Part model, mm, in its own coordinate system. A direction names the side the tool comes from. Give positions to 0.01 mm unless a question says otherwise; leave off trailing zeros. Write each loop counter-clockwise with the first axis right and the second up, starting at its lowest first coordinate (ties: lowest second). Pieces come first, ordered by that corner, then holes.
from build123d import *

# Parameters (mm, degrees)
BOSS_EXTRUDE1_DEPTH = 9.525
SKETCH2_W           = 139.7
SKETCH2_H           = 25.4
CUT_EXTRUDE1_DEPTH  = 503.984538157


with BuildPart() as part:
    # Sketch1 → Boss-Extrude1 (new body)
    with BuildSketch(Plane.XY):
        with BuildLine():
            Line((25.4, 0), (330.2, 0))
            ThreePointArc((330.2, 0), (348.160512242, 7.439487758), (355.6, 25.4))
            Line((355.6, 25.4), (355.6, 330.2))
            ThreePointArc((355.6, 330.2), (348.160512242, 348.160512242), (330.2, 355.6))
            Line((330.2, 355.6), (25.4, 355.6))
            ThreePointArc((25.4, 355.6), (7.439487758, 348.160512242), (0, 330.2))
            Line((0, 330.2), (0, 25.4))
            ThreePointArc((0, 25.4), (7.439487758, 7.439487758), (25.4, 0))
        make_face()
    extrude(amount=BOSS_EXTRUDE1_DEPTH)

    # Sketch2 → Cut-Extrude1 (cut, through all)
    with BuildSketch(Plane(origin=(0, 0, 0), x_dir=(-1, 0, 0), z_dir=(0, 0, -1))):
        with Locations((-177.8, 342.9)):
            Rectangle(SKETCH2_W, SKETCH2_H)
        with Locations((-177.8, 12.7)):
            Rectangle(SKETCH2_W, SKETCH2_H)
    extrude(amount=-CUT_EXTRUDE1_DEPTH, mode=Mode.SUBTRACT)


solid = part.part
1) Saw through at A-A (z = 5.5). Write the cut outline in (x, y).
Check result:
outline: (0, 25.4) arc R25.4 ccw to (25.4, 0) - (107.95, 0) - (107.95, 25.4) - (247.65, 25.4) - (247.65, 0) - (330.2, 0) arc R25.4 ccw to (355.6, 25.4) - (355.6, 330.2) arc R25.4 ccw to (330.2, 355.6) - (247.65, 355.6) - (247.65, 330.2) - (107.95, 330.2) - (107.95, 355.6) - (25.4, 355.6) arc R25.4 ccw to (0, 330.2) - close
2) Drill centre lines: L1, parallel to Y at x = 114.5, z = 8.5; L2, parallel to Y at x = 336.5, z = 3.75. Where is each one in solid material? Low to high.
Check result:
L1: y = 25.4 to 330.2
L2: y = 0.79 to 354.81
3) Saw through at B-B (x = 187.5). Write the cut outline in (y, z) (3 decimals).
Check result:
outline: (25.4, 0) - (330.2, 0) - (330.2, 9.525) - (25.4, 9.525) - close
4) 3-axis set-ups, long thin cutter, end or side, ignore diameter. For faces 5 (the flat face through (107.95, 13, 5)), 6 (the cylindrical face through (7.64, 348.36, 4.7)), 7 (the flat face through (179, 330.2, 5)): which of +Z, -Z, +X, -X, +Y, -Y reach the whole face in a straight line?
Check result:
face 5: +Z, -Z, -Y
face 6: +Z, -Z, -X, +Y
face 7: +Z, -Z, +Y
5) Mould opens along X. For faces 1 (the cylindrical face through (7.24, 7.64, 4.7)), 2 (the flat face through (288, 0, 5)), 3 (the cylindrical face through (348.36, 347.96, 4.7)), 4 (the flat face through (247.65, 343, 5)) say: +X half, -X half, draft (parallel to the pull), parting line (faces both ways), or undercut.
Check result:
face 1: -X half
face 2: draft
face 3: +X half
face 4: undercut
6) Flat gauge pins, fed straight in: P1, Ø3, axis at y = 18, z = 5, coming from the -X side; P2, Ø3, axis at x = 199.5, z = 5, coming from the -Y side; P3, Ø2, axis at x = 71.5, y = 211.5, coming from the -Z side; P4, Ø3, axis at x = 188, z = 3, coming from the +Y side. Where does each tip first touch, or does it go through?
Check result:
P1: stops at x = 0.69
P2: stops at y = 25.4
P3: stops at z = 0
P4: stops at y = 330.2
